Verification items for the finished model (mm, model axes). A direction names the side the tool comes from. Round coordinates to 2 decimals unless told otherwise and drop trailing zeros. Loops run counter-clockwise (first coordinate to the right, second up) from the corner with the lowest first, then second, coordinate; pieces in that order, holes last. Notation, with made-up numbers: M -34.5,66 L 24.5,66 A16 ccw 24.5,95 Z; hole C 79,59.5 d5. An arc over 180 degrees is marked long. One line per item, written item: value.
from build123d import *

# Parameters (mm, degrees)
SKETCH_1_W          = 92
SKETCH_1_H          = 116.5
EXTRUDE_1_DEPTH     = 5
SKETCH_2_W          = 82
SKETCH_2_H          = 5
SKETCH_2_W_2        = 42
EXTRUDE_2_DEPTH     = 23
SKETCH_3_R          = 1.5
CUT_EXTRUDE_1_DEPTH = 129.653427027


with BuildPart() as part:
    # 草圖1 → 填料-伸長1 (new body)
    with BuildSketch(Plane.XY):
        with Locations((0.855675066, -22.881766382)):
            Rectangle(SKETCH_1_W, SKETCH_1_H)
    extrude(amount=EXTRUDE_1_DEPTH)

    # 草圖2 → 填料-伸長2 (add)
    with BuildSketch(Plane.XY.offset(5)):
        with Locations((0.855675066, -78.631766382)):
            Rectangle(SKETCH_2_W, SKETCH_2_H)
        with Locations((20.855675066, 32.868233618)):
            Rectangle(SKETCH_2_W_2, SKETCH_2_H)
    extrude(amount=EXTRUDE_2_DEPTH)

    # 草圖3 → 除料-伸長1 (cut, through all)
    with BuildSketch(Plane.XZ.offset(81.131766382)):
        with Locations(Location((-25.144324934, 18, 0), (0, 0, 270))):
            Circle(SKETCH_3_R)
        with Locations(Location((26.855675066, 18, 0), (0, 0, 270))):
            Circle(SKETCH_3_R)
    extrude(amount=-CUT_EXTRUDE_1_DEPTH, mode=Mode.SUBTRACT)


solid = part.part
(1) Mould release check, pull along X, two halves, no side actions. Record for faces 1 (the face through (21, 30.368, 16)), 2 (the face through (41.856, -79, 16)), 3 (the face through (28.343, -78.667, 18.195)), 4 (the face through (28.343, 32.833, 18.195)): +X half, -X half, draft (parallel to the pull), parting line (faces both ways), or undercut.
Completed:
face 1: draft
face 2: +X half
face 3: undercut
face 4: undercut
(2) Thickness scan on L1, parallel to X at y = -79, z = 18; L2, parallel to X at y = 32.75, z = 18; L3, parallel to Y at x = 31.5, z = 21. Record the ranges inside material, lowest first. Write a range as from..to.
Completed:
L1: x = -40.14..-26.64, -23.64..25.36, 28.36..41.86
L2: x = -0.14..25.36, 28.36..41.86
L3: y = -81.13..-76.13, 30.37..35.37
(3) Sectioned sample at D-D on y = 19.5. Enter the section's corners in (x, z).
Completed:
outline: M -45.14,0 L 46.86,0 L 46.86,5 L -45.14,5 Z
(4) Tool access check on faces 5 (the face through (-40.144, -79, 16)), 6 (the face through (-0.144, 33, 16)), 7 (the face through (41.856, 33, 16)), 8 (the face through (0, -76.132, 16)). Record the directions out of +Z, -Z, +X, -X, +Y, -Y that give a thin tool (end or side, any length) a straight path to the whole face; none if there is none.
Completed:
face 5: +Z, -X, +Y, -Y
face 6: +Z, -X, +Y
face 7: +Z, +X, +Y, -Y
face 8: +Z, +X, -X
(5) Sectioned sample at B-B on z = 11. Enter the section's corners in (x, y), and give its area (3 significant figures).
Completed:
outline: M -40.14,-81.13 L 41.86,-81.13 L 41.86,-76.13 L -40.14,-76.13 Z; M -0.14,30.37 L 41.86,30.37 L 41.86,35.37 L -0.14,35.37 Z
area: 620 mm^2
(6) Sectioned sample at C-C on x = 8.5. Enter the section's corners in (y, z), and give its area (4 significant figures).
Completed:
outline: M -81.13,0 L 35.37,0 L 35.37,28 L 30.37,28 L 30.37,5 L -76.13,5 L -76.13,28 L -81.13,28 Z
area: 812.5 mm^2
(7) Depth check by flat-ended pin: pin 1 Ø7 at (x, z) = (-14.5, 13.5) entering from +Y; pin 2 Ø4 at (y, z) = (-79, 12.5) entering from -X; pin 3 Ø8 at (x, y) = (-31, -39) entering from +Z. Enter the tip coordinate at first touch or a pass-through.
Completed:
pin 1: stops at y = -76.13
pin 2: stops at x = -40.14
pin 3: stops at z = 5
(8) Sectioned sample at A-A on z = 18. Enter the section's corners in (x, y).
Completed:
outline: M -40.14,-81.13 L -26.64,-81.13 L -26.64,-76.13 L -40.14,-76.13 Z; M -23.64,-81.13 L 25.36,-81.13 L 25.36,-76.13 L -23.64,-76.13 Z; M -0.14,30.37 L 25.36,30.37 L 25.36,35.37 L -0.14,35.37 Z; M 28.36,-81.13 L 41.86,-81.13 L 41.86,-76.13 L 28.36,-76.13 Z; M 28.36,30.37 L 41.86,30.37 L 41.86,35.37 L 28.36,35.37 Z
